Input: dimensioned drawing with shaded views. Units: mm. Origin: part minimum x, y, z. Round coordinates to 2 decimals unless told otherwise and drop trailing zeros. Loops run counter-clockwise (first coordinate to the right, second up) from the corner with the lowest first, then second, coordinate; pieces in that order, holes last. Notation, with made-up numbers: (-2.75, 78.5) - (3.25, 78.5) arc R23 ccw to (3.25, 105.5) - close; hole circle Ø1 at (-38, 6.5). An arc over 180 degrees is marked (long way). Answer as CSV lines item,"result".
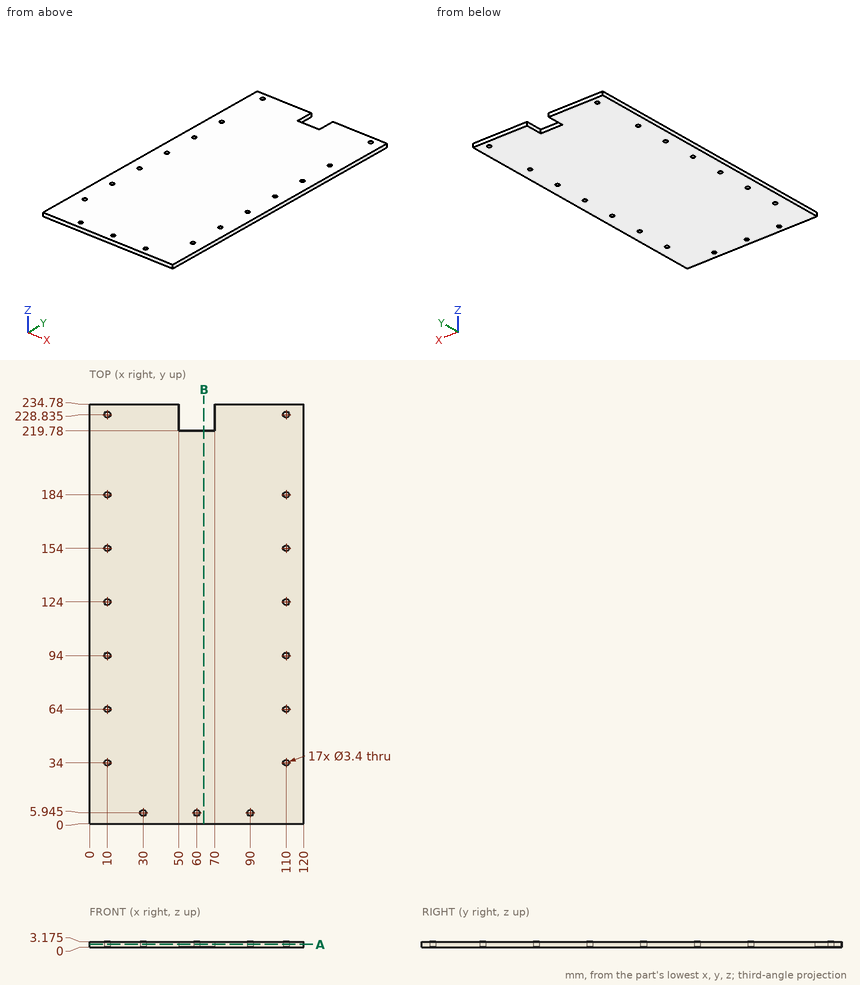
(1) Section A-A (z = 1.6). Give the number of separate pieces and of enclosed holes in the cut face, and give its area (3 significant figures).
Findings below:
separate pieces,"1"
enclosed holes,"17"
area,"27,700 mm2"
(2) Material intervals for line 1 along X through (y, z) = (124, 2.25); line 2 along X through (y, z) = (63, 1.65) (1 decimal), sorted ascending.
Findings below:
line 1,"0 to 8.3, 11.7 to 108.3, 111.7 to 120"
line 2,"0 to 8.6, 11.4 to 108.6, 111.4 to 120"
(3) Section B-B (x = 64). Output: boundary loops of the cut face in (y, z) (3 decimals), and give its area (3 significant figures).
Findings below:
outline,"(0, 0) - (219.78, 0) - (219.78, 3.175) - (0, 3.175) - close"
area,"698 mm2"
